```python
from build123d import *

# Parameters (mm, degrees)
F0_W     = 152.4
F0_H     = 152.4
F1_DEPTH = 63.5
F3_DEPTH = 76.2


with BuildPart() as f1:
    # F0 (on Top) → F1 (new body, symmetric)
    with BuildSketch(Plane.XY):
        Rectangle(F0_W, F0_H)
    extrude(amount=F1_DEPTH, both=True)

    # F2 (on face) → F3 (cut)
    with BuildSketch(Plane.YZ.offset(76.2)):
        with BuildLine():
            Line((76.2, 25.4), (76.2, 50.8))
            ThreePointArc((76.2, 50.8), (63.5, 38.1), (76.2, 25.4))
        make_face()
        with BuildLine():
            ThreePointArc((76.2, 25.4), (85.180256, 29.119744), (88.9, 38.1))
            ThreePointArc((88.9, 38.1), (85.180256, 47.080256), (76.2, 50.8))
            Line((76.2, 50.8), (76.2, 25.4))
        make_face()
    extrude(amount=-F3_DEPTH, mode=Mode.SUBTRACT)


solid = f1.part
```
Source: CAD feature listing. Evaluate the final solid. Frame: model axes, mm. A direction names the side the tool comes from. Coordinates: 2 decimals unless noted, no trailing zeros. Write each loop counter-clockwise with the first axis right and the second up, starting at its lowest first coordinate (ties: lowest second). Pieces come first, ordered by that corner, then holes. Notation, with made-up numbers: (55, 37.5) - (105, 37.5) arc R14 ccw to (105, 54.5) - close; hole circle Ø1 at (7, -37.5). An arc over 180 degrees is marked (long way). Answer as a JSON object with one key per item and string values.
Q1. Material intervals for line 1 (X direction, y = 66, z = 37.5); line 2 (Y direction, x = 70, z = 39), sorted ascending. Write a range as [from, to].
Ans:
{"line 1": "x = [-76.2, 0]", "line 2": "y = [-76.2, 63.53]"}
Q2. Draft query along Z for faces 1 (the flat face through (-1, 1, -63.5)), 2 (the cylindrical face through (38.633, 63.503, 38.379)), 3 (the flat face through (-1, 1, 63.5)), 4 (the flat face through (76.2, -1, 1)). Return one class per face: released by +Z, released by -Z, zero draft, split by the parting line, or undercut.
Ans:
{"face 1": "released by -Z", "face 2": "undercut", "face 3": "released by +Z", "face 4": "zero draft"}
Q3. Set-up query: faces 5 (the flat face through (0, 71, 38)), 6 (the flat face through (-76.2, -1, 1)). Return all of +Z, -Z, +X, -X, +Y, -Y with unobstructed straight access to the full face (end or side cutting, diameter ignored); none if empty.
Ans:
{"face 5": "+X, +Y", "face 6": "+Z, -Z, -X, +Y, -Y"}
Q4. Section query A-A, the plane z = 38.1. Output: boundary loops of the cut face in (x, y), plus the area to 3 significant figures.
Ans:
{"outline": "(-76.2, -76.2) - (76.2, -76.2) - (76.2, 63.5) - (0, 63.5) - (0, 76.2) - (-76.2, 76.2) - close", "area": "22,300 mm2"}
Q5. First-contact query: pin 1 Ø6.5 at (y, z) = (71.5, 40) entering from +X. Flat tip, straight axial feed; report the tip coordinate or a pass-through.
Ans:
{"pin 1": "stops at x = 0"}
